```python
from build123d import *

# Parameters (mm, degrees)
BOSS_EXTRUDE1_DEPTH  = 5
CUT_EXTRUDE1_DEPTH   = 4
CUT_EXTRUDE2_DEPTH   = 29.887713651
M3_CLEARANCE_HOLE1_D = 3.4
FILLET1_R            = 1


with BuildPart() as part:
    # Sketch1 → Boss-Extrude1 (new, symmetric)
    with BuildSketch(Plane(origin=(0, 0, 0), x_dir=(1, 0, 0), z_dir=(0, 1, 0))):
        Polygon((-7.5, 21.5), (7.5, 21.5), (7.5, 3.5), (16.5, 3.5), (16.5, 0), (-16.5, 0), (-16.5, 3.5), (-7.5, 3.5), align=None)
    extrude(amount=BOSS_EXTRUDE1_DEPTH, both=True)

    # Sketch3 → Cut-Extrude1 (cut)
    with BuildSketch(Plane(origin=(0, 5, 0), x_dir=(1, 0, 0), z_dir=(0, 1, 0))):
        with BuildLine():
            Line((4.5, 6), (4.5, 15))
            ThreePointArc((4.5, 15), (0, 19.5), (-4.5, 15))
            Line((-4.5, 15), (-4.5, 6))
            ThreePointArc((-4.5, 6), (0, 1.5), (4.5, 6))
        make_face()
    extrude(amount=-CUT_EXTRUDE1_DEPTH, mode=Mode.SUBTRACT)

    # Sketch4 → Cut-Extrude2 (cut, through all)
    with BuildSketch(Plane(origin=(0, 5, 0), x_dir=(1, 0, 0), z_dir=(0, 1, 0))):
        with BuildLine():
            Line((2.1, 6), (2.1, 15))
            ThreePointArc((2.1, 15), (0, 17.1), (-2.1, 15))
            Line((-2.1, 15), (-2.1, 6))
            ThreePointArc((-2.1, 6), (0, 3.9), (2.1, 6))
        make_face()
    extrude(amount=-CUT_EXTRUDE2_DEPTH, mode=Mode.SUBTRACT)

    # M3 Clearance Hole1 (through all)
    with Locations(Plane(origin=(0, 0, -3.5), x_dir=(-1, 0, 0), z_dir=(0, 0, -1))):
        with Locations((-12, 0), (12, 0)):
            Hole(M3_CLEARANCE_HOLE1_D / 2)

    # Fillet1
    fillet1_edges = [part.edges().sort_by_distance(p)[0] for p in [
        (-7.5, 0, -3.5),
        (7.5, 0, -3.5),
    ]]
    fillet(fillet1_edges, radius=FILLET1_R)


solid = part.part
```
For this review, take the finished solid that the model builds, in its own axes (mm). A direction names the side the tool comes from. Round coordinates to 2 decimals unless told otherwise and drop trailing zeros. Write each loop counter-clockwise with the first axis right and the second up, starting at its lowest first coordinate (ties: lowest second). Pieces come first, ordered by that corner, then holes. Notation, with made-up numbers: (20, -34.75) -> (27, -34.75) arc R22 cw to (27, -13.75) -> close; hole circle Ø7 at (12, 3.5). An arc over 180 degrees is marked (long way). Use one line per item in the form item = value.
1) Tool access review of faces 5 (the flat face through (14, 0, -3.5)), 6 (the flat face through (-2.1, -2, -11)), 7 (the flat face through (-13.44, 1.18, -3.5)), 8 (the flat face through (4.5, 3, -10)): name each direction out of +Z, -Z, +X, -X, +Y, -Y from which nothing blocks a thin tool from reaching the whole face with its end or side.
Found:
face_5 = -Z, +X, +Y, -Y
face_6 = +Y, -Y
face_7 = -Z, -X, +Y, -Y
face_8 = +Y
2) Clearance check with flat-ended pins moving along their axes: pin 1 (4 mm diameter, centred on x = -12, y = 2, fed in from -Z); pin 2 (5 mm diameter, centred on y = 1, z = -12.5, fed in from -X); pin 3 (2.5 mm diameter, centred on x = -0.5, z = -11, fed in from +Y); pin 4 (2 mm diameter, centred on x = 1.5, z = -14, fed in from +Y). State where each tip first meets the part, or that it passes through.
Found:
pin_1 = -3.5
pin_2 = -7.5
pin_3 = through
pin_4 = 1
3) To check wall thickness, follow L1, parallel to X at y = 4.5, z = -8.75; L2, parallel to X at y = -0.25, z = -13.5; L3, parallel to Y at x = -12, z = -0.9. State the ranges of each line that lie inside material, in increasing order. Write a range as from..to.
Found:
L1 = -7.5..-4.5, 4.5..7.5
L2 = -7.5..-2.1, 2.1..7.5
L3 = -5..-1.7, 1.7..5
4) Take a section at C-C, the plane x = 0. Write out the cut boundary in (y, z), and give its area (3 significant figures).
Found:
outline = (-5, -21.5) -> (5, -21.5) -> (5, -19.5) -> (1, -19.5) -> (1, -17.1) -> (-5, -17.1) -> close; (-5, -3.9) -> (1, -3.9) -> (1, -1.5) -> (5, -1.5) -> (5, 0) -> (-5, 0) -> close
area = 63.8 mm2
5) Take a section at A-A, the plane z = -10.25. Write out the cut boundary in (x, y), and give its area (3 significant figures).
Found:
outline = (-7.5, -5) -> (-2.1, -5) -> (-2.1, 1) -> (-4.5, 1) -> (-4.5, 5) -> (-7.5, 5) -> close; (2.1, -5) -> (7.5, -5) -> (7.5, 5) -> (4.5, 5) -> (4.5, 1) -> (2.1, 1) -> close
area = 88.8 mm2
6) Mouldability with a two-part tool opening along Z and no side actions: class faces 1 (the cylindrical face through (-10.38, 0.51, -1.73)), 2 (the cylindrical face through (-7.785, 0.07, -3.801)), 3 (the cylindrical face through (0, -2, -17.1)), 4 (the flat face through (0, 0, 0)) as +Z half, -Z half, draft (parallel to the pull), parting line (faces both ways), or undercut.
Found:
face_1 = draft
face_2 = -Z half
face_3 = undercut
face_4 = +Z half
7) Take a section at D-D, the plane x = 12. Write out the cut boundary in (y, z).
Found:
outline = (-5, -3.5) -> (-1.7, -3.5) -> (-1.7, 0) -> (-5, 0) -> close; (1.7, -3.5) -> (5, -3.5) -> (5, 0) -> (1.7, 0) -> close
8) Take a section at B-B, the plane y = 3. Write out the cut boundary in (x, z).
Found:
outline = (-16.5, -3.5) -> (-8.5, -3.5) arc R1 cw to (-7.5, -4.5) -> (-7.5, -21.5) -> (7.5, -21.5) -> (7.5, -4.5) arc R1 cw to (8.5, -3.5) -> (16.5, -3.5) -> (16.5, 0) -> (-16.5, 0) -> close; hole (-4.5, -15) arc R4.5 ccw to (4.5, -15) -> (4.5, -6) arc R4.5 ccw to (-4.5, -6) -> close
